Geometry: see drawing. Coordinates: mm, zero at the bounding-box minimum. Coordinates: 2 decimals unless noted, no trailing zeros. Write each loop counter-clockwise with the first axis right and the second up, starting at its lowest first coordinate (ties: lowest second). Pieces come first, ordered by that corner, then holes. Notation, with made-up numbers: (38, 58) - (65, 58) arc R28 ccw to (65, 87) - close; hole circle Ø6 at (5.25, 17.25). An arc over 180 degrees is marked (long way). One line per question, with ' | ' between items. Start each with the question number.
1) Section query B-B on z = 47.5. Return loops of the section in (x, y).
2) Section query A-A on y = 2. Return loops of the section in (x, z), and give its area (3 significant figures).
3) Section query C-C on x = 14.5. Return loops of the section in (y, z), and give its area (3 significant figures).
4) Line query: line 1 (Z direction, x = 5, y = 0.6); line 2 (X direction, y = 0.95, z = 14.5); line 3 (Z direction, x = 45.5, y = 2.6). Output: solid intervals per line, ascending.
5) First-contact query: P1, Ø3.5, axis at x = 5.5, z = 5.5, coming from the -Y side; P2, Ø2.5, axis at x = 45.5, z = 54.5, coming from the +Y side; P3, Ø0.9, axis at y = 1.5, z = 35, coming from the -X side; P4, Ø0.9, axis at x = 22, y = 2, coming from the +Z side. Flat tips, straight axial feed; report the tip coordinate or a pass-through.
6) Draft query along Y for the marked faces 1 and 2. Return one class per face: released by +Y, released by -Y, zero draft, split by the parting line, or undercut.
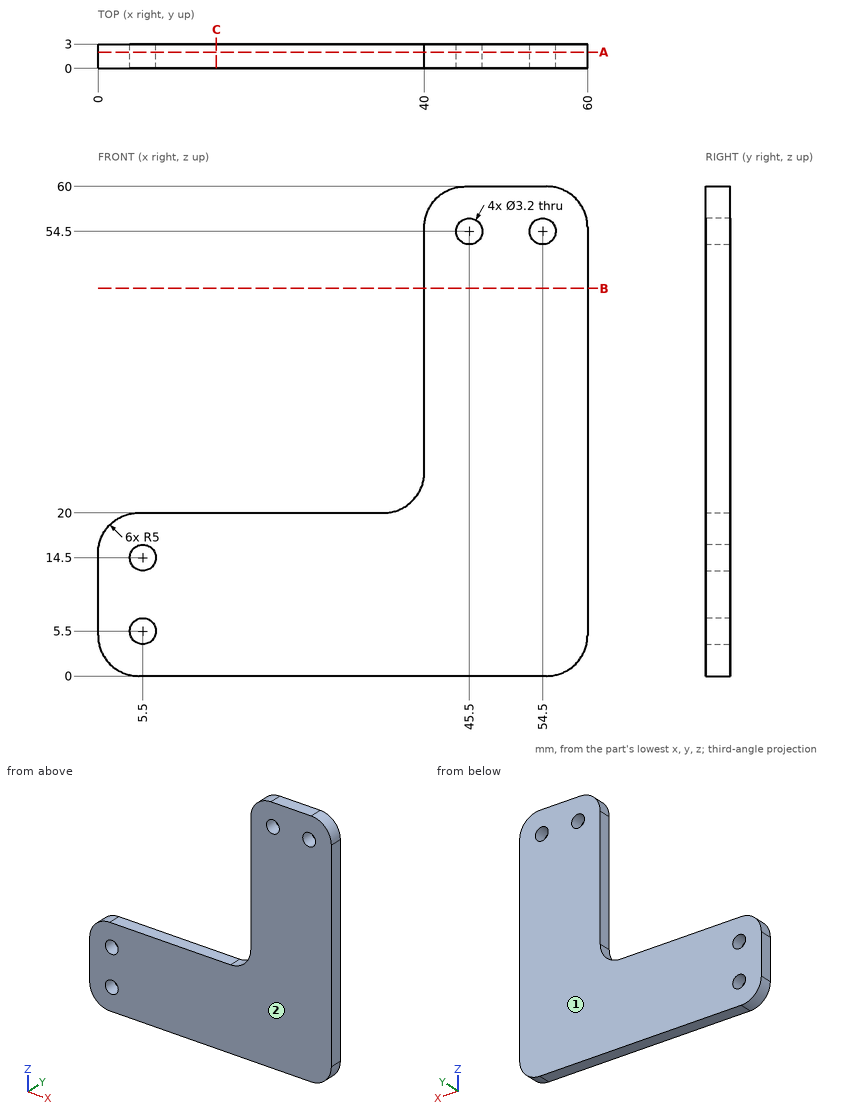
Answer key:
1) outline: (40, 0) - (60, 0) - (60, 3) - (40, 3) - close
2) outline: (0, 5) arc R5 ccw to (5, 0) - (55, 0) arc R5 ccw to (60, 5) - (60, 55) arc R5 ccw to (55, 60) - (45, 60) arc R5 ccw to (40, 55) - (40, 25) arc R5 cw to (35, 20) - (5, 20) arc R5 ccw to (0, 15) - close; hole circle Ø3.2 at (5.5, 5.5); hole circle Ø3.2 at (5.5, 14.5); hole circle Ø3.2 at (45.5, 54.5); hole circle Ø3.2 at (54.5, 54.5) | area: 1,950 mm²
3) outline: (0, 0) - (3, 0) - (3, 20) - (0, 20) - close | area: 60.0 mm²
4) line 1: 0 to 3.98, 7.02 to 12.98, 16.02 to 20 | line 2: 0 to 3.9, 7.1 to 60 | line 3: 0 to 52.9, 56.1 to 60
5) P1: y = 0 | P2: through | P3: x = 40 | P4: z = 20
6) face 1: released by +Y | face 2: released by -Y
